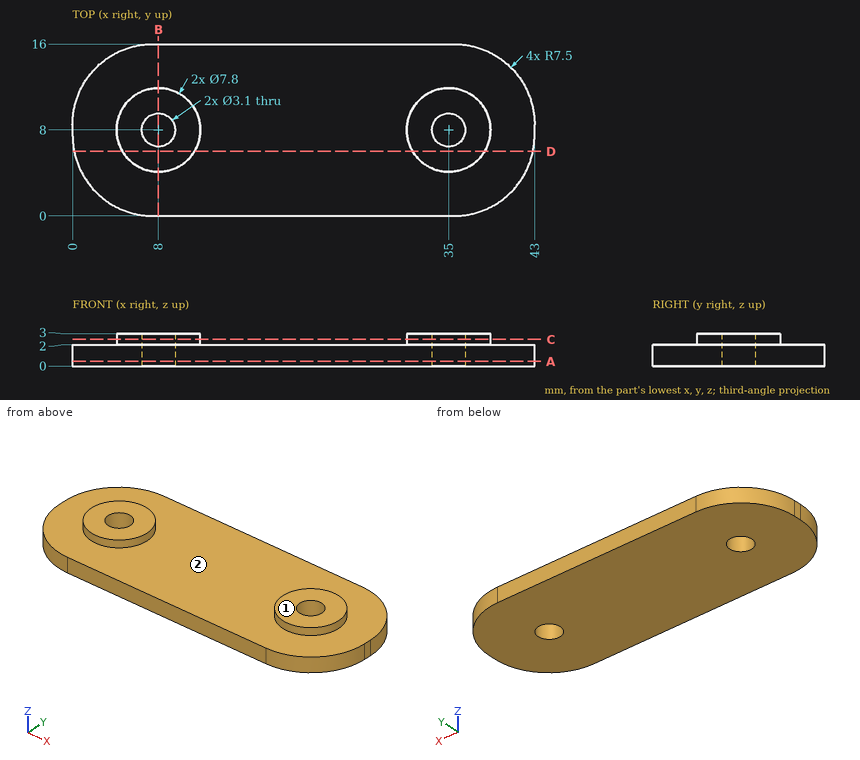
The figure shows three views and two pictorial views of one solid part (mm, origin at its lowest corner). Answer the questions. A direction names the side the tool comes from. Coordinates: 2 decimals unless noted, no trailing zeros. Loops run counter-clockwise (first coordinate to the right, second up) from the corner with the lowest first, then second, coordinate; pieces in that order, holes last. Notation, with made-up numbers: (43.25, 38.25) -> (47.25, 38.25) arc R25 ccw to (47.25, 51.25) -> close; hole circle Ø10 at (74.5, 78). An arc over 180 degrees is marked (long way). Return JSON: item names as keys, results as strings. Group by question number.
(1) A cutting plane is placed at A-A on z = 0.45. Write down the section's boundary in (x, y).
(2) Given pin 1 Ø1.5 at (y, z) = (2, 1.5) entering from -X; pin 2 Ø8 at (x, y) = (24.5, 10.5) entering from +Z; pin 3 Ø1.9 at (x, y) = (8, 8) entering from +Z; pin 4 Ø1.5 at (y, z) = (4, 1) entering from +X, each flat-ended and moving along its own axis, determine where each tip first touches the part or whether it passes through.
(3) A cutting plane is placed at B-B on x = 8. Write down the section's boundary in (y, z).
(4) A cutting plane is placed at D-D on y = 6. Write down the section's boundary in (x, z).
(5) A cutting plane is placed at C-C on z = 2.5. Write down the section's boundary in (x, y).
(6) Find the intervals of material crossed by probe 1 along Y at (x, z) = (8, 0.95); probe 2 along Y at (x, z) = (8, 2.4); probe 3 along X at (y, z) = (7.5, 1.65), in increasing order. Write a range as from..to.
(7) Which of the six approach directions +Z, -Z, +X, -X, +Y, -Y give full straight-line access (tool end or side, diameter ignored) to the marked faces 1 and 2?
The answers:
{
 "1": {"outline": "(0, 7.5) arc R7.5 ccw to (7.5, 0) -> (35.5, 0) arc R7.5 ccw to (43, 7.5) -> (43, 8.5) arc R7.5 ccw to (35.5, 16) -> (7.5, 16) arc R7.5 ccw to (0, 8.5) -> close; hole circle Ø3.1 at (8, 8); hole circle Ø3.1 at (35, 8)"},
 "2": {"pin 1": "stops at x = 1.7", "pin 2": "stops at z = 2", "pin 3": "passes through", "pin 4": "stops at x = 42.48"},
 "3": {"outline": "(0, 0) -> (6.45, 0) -> (6.45, 3) -> (4.1, 3) -> (4.1, 2) -> (0, 2) -> close; (9.55, 0) -> (16, 0) -> (16, 2) -> (11.9, 2) -> (11.9, 3) -> (9.55, 3) -> close"},
 "4": {"outline": "(0.15, 0) -> (42.85, 0) -> (42.85, 2) -> (38.35, 2) -> (38.35, 3) -> (31.65, 3) -> (31.65, 2) -> (11.35, 2) -> (11.35, 3) -> (4.65, 3) -> (4.65, 2) -> (0.15, 2) -> close"},
 "5": {"outline": "circle Ø7.8 at (8, 8); circle Ø7.8 at (35, 8); hole circle Ø3.1 at (8, 8); hole circle Ø3.1 at (35, 8)"},
 "6": {"probe 1": "y = 0..6.45, 9.55..16", "probe 2": "y = 4.1..6.45, 9.55..11.9", "probe 3": "x = 0..6.53, 9.47..33.53, 36.47..43"},
 "7": {"face 1": "+Z, +X, -X, +Y, -Y", "face 2": "+Z"}
}
